Work out the finished part from the listing and answer in its coordinate system (mm). Face numbers are marked on the shaded views. A direction names the side the tool comes from. Give positions to 0.01 mm unless a question says otherwise; leave off trailing zeros. Loops run counter-clockwise (first coordinate to the right, second up) from the corner with the lowest first, then second, coordinate; pieces in that order, holes last. Notation, with made-up numbers: (65, 88.5) - (124, 88.5) arc R27 cw to (124, 116.5) - close; hole circle Ø6 at (47, 87). An arc over 180 degrees is marked (long way). One line per question, with ' | ' between items.
from build123d import *

# Parameters (mm, degrees)
BOSS_EXTRUDE1_DEPTH = 2
SKETCH3_R           = 2.375
SKETCH3_R_2         = 2.372845421
BOSS_EXTRUDE3_DEPTH = 5


with BuildPart() as part:
    # Sketch1 → Boss-Extrude1 (new body)
    with BuildSketch(Plane(origin=(0, 0, 0), x_dir=(1, 0, 0), z_dir=(0, 1, 0))):
        Polygon((-22, 8.714285714), (-22, -8.714285714), (22, -8.714285714), (22, 8.714285714), (11.25, 33.285714286), (-11.1, 33.285714286), align=None)
    extrude(amount=BOSS_EXTRUDE1_DEPTH)

    # Sketch3 → Boss-Extrude3 (add)
    with BuildSketch(Plane.XZ):
        with Locations(Location((-10, -3.285714286, 0), (0, 0, 270))):
            Circle(SKETCH3_R)
        with Locations(Location((-9.991570168, -28.264481029, 0), (0, 0, 270))):
            Circle(SKETCH3_R_2)
        with Locations(Location((10, -28.285714286, 0), (0, 0, 270))):
            Circle(SKETCH3_R)
        with Locations(Location((10, -3.285714286, 0), (0, 0, 270))):
            Circle(SKETCH3_R)
    extrude(amount=BOSS_EXTRUDE3_DEPTH)


solid = part.part
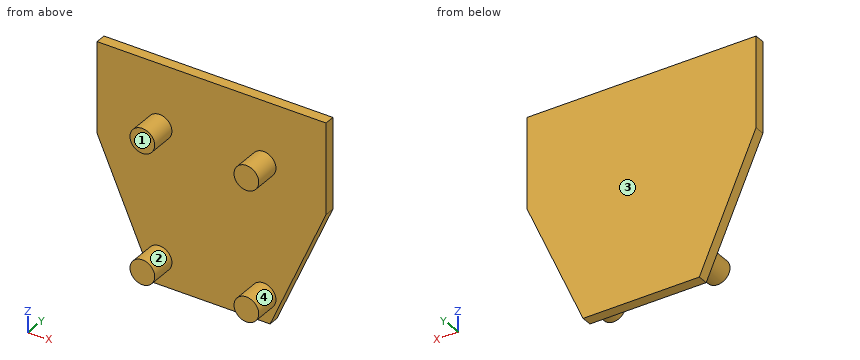
1. Find section A-A on x = 10. Write down the section's boundary in (y, z), then the cut area to 4 significant figures.
Evaluation:
outline: (-5, -30.66) - (0, -30.66) - (0, -33.29) - (2, -33.29) - (2, 8.71) - (0, 8.71) - (0, -0.91) - (-5, -0.91) - (-5, -5.66) - (0, -5.66) - (0, -25.91) - (-5, -25.91) - close | area: 131.5 mm2
2. Find section B-B on y = -1.75. Write down the section's boundary in (x, z) (3 decimals).
Evaluation:
outline: circle Ø4.75 at (-10, -3.286); circle Ø4.746 at (-9.992, -28.264); circle Ø4.75 at (10, -28.286); circle Ø4.75 at (10, -3.286)
3. Which of the six approach directions +Z, -Z, +X, -X, +Y, -Y give full straight-line access (tool end or side, diameter ignored) to the marked faces 3 and 4?
Evaluation:
face 3: +Z, -Z, +X, -X, +Y | face 4: -Y
4. Determine the mould class of the marked faces 1 and 2 for opening direction Z: +Z half, -Z half, draft (parallel to the pull), parting line (faces both ways), or undercut.
Evaluation:
face 1: draft | face 2: undercut
5. A flat-ended cylindrical pin translates along its axis: pin 1 (10 mm diameter, centred on x = -4, z = -12, fed in from -Y). Find the tip coordinate at first contact, or state that the pin passes through.
Evaluation:
pin 1: y = 0
6. Consider L1, parallel to Y at x = -7.5, z = -26.5; L2, parallel to X at y = -2, z = -29.5; L3, parallel to X at y = -3.25, z = -1.5. Determine where each line is inside the solid, lowest interval first.
Evaluation:
L1: 0 to 2 | L2: -12.02 to -7.97, 7.96 to 12.04 | L3: -11.57 to -8.43, 8.43 to 11.57
7. Find section D-D on x = 5. Write down the section's boundary in (y, z).
Evaluation:
outline: (0, -33.29) - (2, -33.29) - (2, 8.71) - (0, 8.71) - close
8. Find section C-C on z = -3. Write down the section's boundary in (x, y).
Evaluation:
outline: (-22, 0) - (-12.36, 0) - (-12.36, -5) - (-7.64, -5) - (-7.64, 0) - (7.64, 0) - (7.64, -5) - (12.36, -5) - (12.36, 0) - (22, 0) - (22, 2) - (-22, 2) - close
